from build123d import *

# Parameters (mm, degrees)
F1_DEPTH      = 20
F3_R          = 1.75
F4_DEPTH      = 40.001
F3_R_2        = 3
F5_DEPTH      = 25
F6_W          = 160
F6_H          = 10
F7_DEPTH      = 20.001
F9_DEPTH      = 80.001
F9_DEPTH_BACK = 80.001


with BuildPart() as f1:
    # F0 (on Front) → F1 (new body)
    with BuildSketch(Plane.XZ):
        with BuildLine():
            Line((50, 41), (5, 41))
            Line((5, 41), (-5, 41))
            Line((-5, 41), (-50, 41))
            Line((-50, 41), (-80, 21))
            Line((-80, 21), (-80, 5))
            Line((-80, 5), (-38.5, 5))
            Line((-38.5, 5), (-38.5, 30.5))
            ThreePointArc((-38.5, 30.5), (-38.3535533906, 30.8535533906), (-38, 31))
            Line((-38, 31), (-28.5, 31))
            Line((-28.5, 31), (-28.5, 34))
            ThreePointArc((-28.5, 34), (-28.3535533906, 34.3535533906), (-28, 34.5))
            Line((-28, 34.5), (-19, 34.5))
            ThreePointArc((-19, 34.5), (-18.6464466094, 34.3535533906), (-18.5, 34))
            Line((-18.5, 34), (-18.5, 31))
            Line((-18.5, 31), (0, 31))
            Line((0, 31), (18.5, 31))
            Line((18.5, 31), (18.5, 34))
            ThreePointArc((18.5, 34), (18.6464466094, 34.3535533906), (19, 34.5))
            Line((19, 34.5), (28, 34.5))
            ThreePointArc((28, 34.5), (28.3535533906, 34.3535533906), (28.5, 34))
            Line((28.5, 34), (28.5, 31))
            Line((28.5, 31), (38, 31))
            ThreePointArc((38, 31), (38.3535533906, 30.8535533906), (38.5, 30.5))
            Line((38.5, 30.5), (38.5, 5))
            Line((38.5, 5), (80, 5))
            Line((80, 5), (80, 21))
            Line((80, 21), (50, 41))
        make_face()
    extrude(amount=-F1_DEPTH)

    # F3 (on offset) → F4 (cut, through all)
    with BuildSketch(Plane.XY.offset(45)):
        with Locations((-66.75, 10)):
            Circle(F3_R)
        with Locations((66.75, 10)):
            Circle(F3_R)
    extrude(amount=-F4_DEPTH, mode=Mode.SUBTRACT)

    # F3 (on offset) → F5 (cut)
    with BuildSketch(Plane.XY.offset(45)):
        with Locations((-66.75, 10)):
            Circle(F3_R_2)
        with Locations((-66.75, 10)):
            Circle(F3_R, mode=Mode.SUBTRACT)
        with Locations((66.75, 10)):
            Circle(F3_R_2)
        with Locations((66.75, 10)):
            Circle(F3_R, mode=Mode.SUBTRACT)
    extrude(amount=-F5_DEPTH, mode=Mode.SUBTRACT)

    # F6 (on Front) → F7 (cut, through all)
    with BuildSketch(Plane.XZ):
        with Locations((0, 10)):
            Rectangle(F6_W, F6_H)
    extrude(amount=-F7_DEPTH, mode=Mode.SUBTRACT)

    # F8 (on Right) → F9 (cut, two sides)
    with BuildSketch(Plane.YZ) as f9_sk:
        with BuildLine():
            ThreePointArc((4.4999439066, 15), (2.734050334, 15.7303616499), (1.999949516, 17.4947040879))
            Line((1.999949516, 17.4947040879), (1.9893576917, 22.4946928692))
            ThreePointArc((1.9893576917, 22.4946928692), (1.4447268651, 24.2275058154), (0, 25.3284271247))
            Line((0, 25.3284271247), (0, 15))
            Line((0, 15), (2.0052342213, 15))
            Line((2.0052342213, 15), (4.4999439066, 15))
        make_face()
    extrude(amount=-F9_DEPTH, mode=Mode.SUBTRACT)
    extrude(f9_sk.sketch, amount=F9_DEPTH_BACK, mode=Mode.SUBTRACT)


solid = f1.part
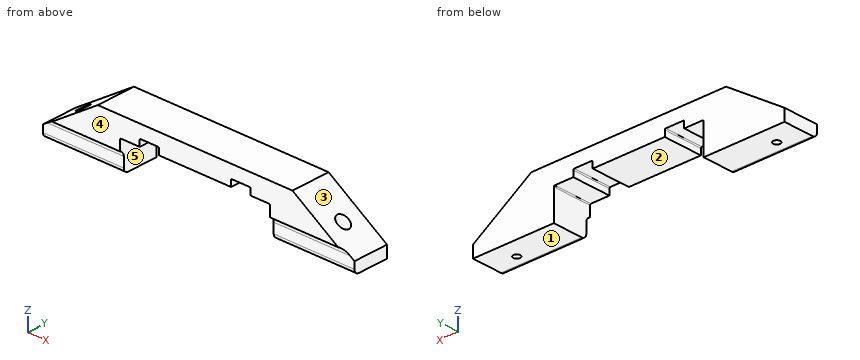
Source: CAD feature listing. Evaluate the final solid. Frame: model axes, mm. Face numbers are marked on the shaded views. A direction names the side the tool comes from. Round coordinates to 2 decimals unless told otherwise and drop trailing zeros. Write each loop counter-clockwise with the first axis right and the second up, starting at its lowest first coordinate (ties: lowest second). Pieces come first, ordered by that corner, then holes. Notation, with made-up numbers: (68.5, 52.5) - (99.5, 52.5) arc R19 cw to (99.5, 58.5) - close; hole circle Ø2 at (68.25, 69.5). An arc over 180 degrees is marked (long way). Use CSV: the item, a comma, the result in double quotes. Start each with the question number.
(1) Cut plane D-D, the plane x = -33.5. Return loops of the section in (y, z), and give its area (3 significant figures).
(2) Cut plane B-B, the plane x = 43. Return loops of the section in (y, z).
(3) Material intervals for probe 1 along Y at (x, z) = (-66.75, 28.5); probe 2 along X at (y, z) = (9.5, 24.75) (3 decimals); probe 3 along X at (y, z) = (11.25, 24.5), sorted ascending. Write a range as [from, to].
(4) Set-up query: the marked faces 4 and 5. Return all of +Z, -Z, +X, -X, +Y, -Y with unobstructed straight access to the full face (end or side cutting, diameter ignored); none if empty.
(5) Mould query, pull axis X, two halves, no side actions, for the marked faces 1, 2 and 3. Classes: pulls with the +X half, pulls with the -X half, needs draft (parallel to the pull), parting line crosses it, or undercut.
(6) Cut plane A-A, the plane x = -66.75. Return loops of the section in (y, z), and give its area (3 significant figures).
(7) First-contact query: pin 1 Ø1.5 at (y, z) = (6, 32) entering from +X (3 decimals); pin 2 Ø1.5 at (y, z) = (12, 37.5) entering from -X (3 decimals); pin 3 Ø2 at (x, y) = (-19, 15.5) entering from -Z; pin 4 Ø5 at (x, z) = (-9.5, 27) entering from -Y. Flat tips, straight axial feed; report the tip coordinate or a pass-through.
(8) Cut plane C-C, the plane y = 10. Give the number of separate pieces and of enclosed holes in the cut face, and give its area (3 significant figures).
Geometry says:
1,outline,"(0, 31) - (20, 31) - (20, 41) - (0, 41) - close"
1,area,"200 mm²"
2,outline,"(0, 25.33) arc R3 cw to (1.99, 22.49) - (2, 17.49) arc R2.5 ccw to (4.5, 15) - (20, 15) - (20, 41) - (0, 41) - close"
3,probe 1,"[0, 7], [13, 20]"
3,probe 2,"[-74.375, -69.708], [-63.792, -38.5], [38.5, 63.792], [69.708, 74.375]"
3,probe 3,"[-74.75, -69.48], [-64.02, -38.5], [38.5, 64.02], [69.48, 74.75]"
4,face 4,"+Z, -Z, +X, -X, -Y"
4,face 5,"-Z, +Y, -Y"
5,face 1,"needs draft"
5,face 2,"undercut"
5,face 3,"pulls with the +X half"
6,outline,"(0, 25.33) arc R3 cw to (1.99, 22.49) - (2, 17.49) arc R2.5 ccw to (4.5, 15) - (8.25, 15) - (8.25, 20) - (7, 20) - (7, 29.83) - (0, 29.83) - close; (11.75, 15) - (20, 15) - (20, 29.83) - (13, 29.83) - (13, 20) - (11.75, 20) - close"
6,area,"200 mm²"
7,pin 1,"x = 64.625"
7,pin 2,"x = -56.375"
7,pin 3,"z = 31"
7,pin 4,"through"
8,separate pieces,"3"
8,enclosed holes,"0"
8,area,"2,110 mm²"
